Design review of the part built by this model. Coordinates are the model's own, in mm. A direction names the side the tool comes from. Round coordinates to 2 decimals unless told otherwise and drop trailing zeros. Loops run counter-clockwise (first coordinate to the right, second up) from the corner with the lowest first, then second, coordinate; pieces in that order, holes last. Notation, with made-up numbers: (44, 10) - (98, 10) arc R17 cw to (98, 26) - close; hole circle Ø2 at (85, 70). An arc over 180 degrees is marked (long way). Return JSON: item names as keys, results as strings. Group by question number.
(1) We need section B-B, the plane x = 5. Write out the cut boundary in (y, z), and give its area (3 significant figures).
(2) For faces 1 (the flat face through (28, 9, -5)), 2 (the flat face through (28, 0, -5)), list the 3-axis set-ups (+Z, -Z, +X, -X, +Y, -Y) from which the entire face can be reached by the end or side of a thin tool; tool diameter is ignored.
(3) Wall thickness on L1, parallel to X at y = 0.4, z = -5; L2, parallel to X at y = 5, z = -0.6; L3, parallel to Z at x = 17, y = 4.25: over which ranges is each line inside the solid? List them lowest first. Write a range as [from, to].
(4) We need section D-D, the plane y = 5. Write out the cut boundary in (x, z).
(5) The part is to be moulded in two halves that separate along X. For faces 3 (the cylindrical face through (12.42, 6.18, -0.51)), 4 (the flat face through (28, 1, -5)), 5 (the flat face through (0, 4.9, -9.4)), say which applies: pulls with the +X half, pulls with the -X half, needs draft (parallel to the pull), parting line crosses it, or undercut.
(6) We need section A-A, the plane y = 8.5. Write out the cut boundary in (x, z), and give its area (3 significant figures).
(7) We need section C-C, the plane z = -7.75. Write out the cut boundary in (x, y).
Autodesk Inventor part; units mm, degrees
ref_plane "YZ Plane" through (0, 0, 0) normal (1, 0, 0) x (0, 1, 0)
ref_plane "XZ Plane" through (0, 0, 0) normal (0, 1, 0) x (-1, 0, 0)
ref_plane "XY Plane" through (0, 0, 0) normal (0, 0, 1) x (1, 0, 0)
sketch "スケッチ1" plane through (0, 0, 0) normal (1, 0, 0) x (0, 1, 0)
  line L0 (0, 0) -> (10, 0)
  line L1 (10, 0) -> (10, -10)
  line L2 (10, -10) -> (0, -10)
  line L3 (0, -10) -> (0, 0)
  line L4 (1, -1) -> (9, -1)
  line L5 (9, -1) -> (9, -9)
  line L6 (9, -9) -> (1, -9)
  line L7 (1, -9) -> (1, -1)
  dimension "d0" = 10
  dimension "d1" = 10
  dimension "d2" = 8
  dimension "d3" = 8
  dimension "d4" = 1
  dimension "d5" = 1
extrude "押し出し1" add sketch "スケッチ1" along normal blind 57
sketch "スケッチ2" plane through (0, 10, 0) normal (0, 1, 0) x (1, 0, 0)
  line L0 (0, 9) -> (0, 1)
  line L1 (0, 5) -> (120, 5)
  line L2 (57, 10) -> (57, 0)
  point P0 (0, 0)
  point P1 (5, 5)
  point P2 (52, 5)
  dimension "d8" = 5
  dimension "d9" = 5
hole "穴1" at (5, 10, -5) at (52, 10, -5) direction (0, -1, 0) diameter 3.2 end through all
sketch "スケッチ3" plane through (0, 0, 0) normal (0, 0, 1) x (1, 0, 0)
  line L0 (0, 0) -> (0, 10)
  line L1 (0, 5) -> (57, 5)
  line L2 (57, 0) -> (57, 10)
  point P0 (13.5, 5)
  point P1 (43.5, 5)
  point P2 (28.5, 5)
  dimension "d17" = 15
  dimension "d18" = 15
hole "穴2" at (13.5, 5, 0) at (43.5, 5, 0) direction (0, 0, -1) diameter 3.2 end through all
properties part number "link4_pipe1" material "アルミニウム 6061"
Solutions:
{
 "1": {"outline": "(0, -10) - (10, -10) - (10, -6.6) - (9, -6.6) - (9, -9) - (1, -9) - (1, -6.6) - (0, -6.6) - close; (0, -3.4) - (1, -3.4) - (1, -1) - (9, -1) - (9, -3.4) - (10, -3.4) - (10, 0) - (0, 0) - close", "area": "29.6 mm^2"},
 "2": {"face 1": "+X, -X", "face 2": "+Z, -Z, +X, -X, -Y"},
 "3": {"L1": "[0, 3.4], [6.6, 50.4], [53.6, 57]", "L2": "[0, 11.9], [15.1, 41.9], [45.1, 57]", "L3": "[-10, -9], [-1, 0]"},
 "4": {"outline": "(0, -10) - (11.9, -10) - (11.9, -9) - (0, -9) - close; (0, -1) - (11.9, -1) - (11.9, 0) - (0, 0) - close; (15.1, -10) - (41.9, -10) - (41.9, -9) - (15.1, -9) - close; (15.1, -1) - (41.9, -1) - (41.9, 0) - (15.1, 0) - close; (45.1, -10) - (57, -10) - (57, -9) - (45.1, -9) - close; (45.1, -1) - (57, -1) - (57, 0) - (45.1, 0) - close"},
 "5": {"face 3": "undercut", "face 4": "needs draft", "face 5": "pulls with the -X half"},
 "6": {"outline": "(0, -10) - (57, -10) - (57, -9) - (0, -9) - close; (0, -1) - (57, -1) - (57, 0) - (0, 0) - close", "area": "114 mm^2"},
 "7": {"outline": "(0, 0) - (57, 0) - (57, 1) - (0, 1) - close; (0, 9) - (57, 9) - (57, 10) - (0, 10) - close"}
}
